from build123d import *

# Parameters (mm, degrees)
F0_W     = 76.2
F0_H     = 76.2
F1_DEPTH = 127
F2_R     = 12.7
F3_DEPTH = 76.201
F4_SIZE  = 5.08
F5_R     = 5.08
F7_D     = 6.35


with BuildPart() as f1:
    # F0 (on Top) → F1 (new body)
    with BuildSketch(Plane.XY):
        Rectangle(F0_W, F0_H)
    extrude(amount=F1_DEPTH)

    # F2 (on face) → F3 (cut, through all)
    with BuildSketch(Plane.XZ.offset(38.1)):
        with Locations((0, 63.5)):
            Circle(F2_R)
    extrude(amount=-F3_DEPTH, mode=Mode.SUBTRACT)

    # F4
    f4_edges = [f1.edges().sort_by_distance(p)[0] for p in [
        (-12.7, -38.1, 63.5),
        (-12.7, 38.1, 63.5),
    ]]
    chamfer(f4_edges, length=F4_SIZE)

    # F5
    f5_edges = [f1.edges().sort_by_distance(p)[0] for p in [
        (0, -38.1, 127),
        (38.1, 0, 127),
        (0, 38.1, 127),
        (-38.1, 0, 127),
        (-38.1, 0, 0),
        (38.1, 0, 0),
        (0, 38.1, 0),
        (0, -38.1, 0),
        (38.1, -38.1, 63.5),
        (38.1, 38.1, 63.5),
        (-38.1, 38.1, 63.5),
        (-38.1, -38.1, 63.5),
    ]]
    fillet(f5_edges, radius=F5_R)

    # F7 (through all)
    with Locations(Plane.XY.offset(127)):
        with Locations((0, 0)):
            Hole(F7_D / 2)


solid = f1.part
Geometry: final body of the model. Coordinates: model frame, mm. Coordinates: 2 decimals unless noted, no trailing zeros. Order: outer loops, then holes, each group sorted by start corner. A loop starts at its lowest first (then second) coordinate and runs counter-clockwise, first axis right, second up.
(1) Material intervals for probe 1 along X at (y, z) = (0, 14) (3 decimals); probe 2 along Z at (x, y) = (0, -10.5), sorted ascending.
(2) Section query A-A (x = 0). Return the cut outline in (y, z) (3 decimals).
(3) Draft query along Y for faces 1 (the face through (0.462, 36.572, 125.551)), 2 (the face through (-36.651, 0.462, 125.472)), 3 (the face through (0.69, -3.1, 25.25)). Return one class per face: pulls with the +Y half, pulls with the -Y half, needs draft (parallel to the pull), parting line crosses it, or undercut.
(4) Section query B-B (y = 26). Return the cut outline in (x, z), plus the area to 3 significant figures.
(5) First-contact query: pin 1 (5 mm diameter, centred on x = 0, y = 0, fed in from +Z). Flat tip, straight axial feed; report the tip coordinate or a pass-through.
(6) Section query C-C (z = 63.5). Return the cut outline in (x, y).
(7) Section query D-D (y = 0). Return the cut outline in (x, z) (3 decimals), plus the area to 3 significant figures.
Solution:
1. probe 1: x = -38.1 to -3.175, 3.175 to 38.1
1. probe 2: z = 0 to 50.8, 76.2 to 127
2. outline: (-38.1, 5.08) arc R5.08 ccw to (-33.02, 0) - (-3.175, 0) - (-3.175, 50.8) - (-33.02, 50.8) - (-38.1, 45.72) - close; (-38.1, 81.28) - (-33.02, 76.2) - (-3.175, 76.2) - (-3.175, 127) - (-33.02, 127) arc R5.08 ccw to (-38.1, 121.92) - close; (3.175, 0) - (33.02, 0) arc R5.08 ccw to (38.1, 5.08) - (38.1, 45.72) - (33.02, 50.8) - (3.175, 50.8) - close; (3.175, 76.2) - (33.02, 76.2) - (38.1, 81.28) - (38.1, 121.92) arc R5.08 ccw to (33.02, 127) - (3.175, 127) - close
3. face 1: pulls with the +Y half
3. face 2: needs draft
3. face 3: undercut
4. outline: (-38.1, 5.08) arc R5.08 ccw to (-33.02, 0) - (33.02, 0) arc R5.08 ccw to (38.1, 5.08) - (38.1, 121.92) arc R5.08 ccw to (33.02, 127) - (-33.02, 127) arc R5.08 ccw to (-38.1, 121.92) - close; hole circle Ø25.4 at (0, 63.5)
4. area: 9,150 mm2
5. pin 1: passes through
6. outline: (-38.1, -33.02) arc R5.08 ccw to (-33.02, -38.1) - (-17.78, -38.1) - (-12.7, -33.02) - (-12.7, 33.02) - (-17.78, 38.1) - (-33.02, 38.1) arc R5.08 ccw to (-38.1, 33.02) - close; (12.7, -33.02) - (17.78, -38.1) - (33.02, -38.1) arc R5.08 ccw to (38.1, -33.02) - (38.1, 33.02) arc R5.08 ccw to (33.02, 38.1) - (17.78, 38.1) - (12.7, 33.02) - close
7. outline: (-38.1, 5.08) arc R5.08 ccw to (-33.02, 0) - (-3.175, 0) - (-3.175, 51.203) arc R12.7 cw to (-3.175, 75.797) - (-3.175, 127) - (-33.02, 127) arc R5.08 ccw to (-38.1, 121.92) - close; (3.175, 0) - (33.02, 0) arc R5.08 ccw to (38.1, 5.08) - (38.1, 121.92) arc R5.08 ccw to (33.02, 127) - (3.175, 127) - (3.175, 75.797) arc R12.7 cw to (3.175, 51.203) - close
7. area: 8,500 mm2
